Model file for the job. Use its own axes, mm. A direction names the side the tool comes from. Round coordinates to 2 decimals unless told otherwise and drop trailing zeros. Loops run counter-clockwise (first coordinate to the right, second up) from the corner with the lowest first, then second, coordinate; pieces in that order, holes last. Notation, with made-up numbers: M 9.25,14 L 68.25,14 A29 cw 68.25,45 Z; hole C 75.25,-17.75 d11. An arc over 180 degrees is marked long. Use a Markdown table: item, result. Add a question column.
Q1. Pin check, flat tips, straight feed: pin 1 (3 mm diameter, centred on x = -3, y = 5, fed in from +Z); pin 2 (0.5 mm diameter, centred on x = -1.5, y = 5, fed in from +Z); pin 3 (1.5 mm diameter, centred on x = -3.5, z = 1, fed in from -Y). Stop position of each tip, or through.
Q2. Mould opens along X. For faces 3 (the face through (0, 0, 0)), 4 (the face through (4, 4, 2.8)), 5 (the face through (-2.17, -9.76, 1.49)), 6 (the face through (4.65, -2.85, 2.75)) say: +X half, -X half, draft (parallel to the pull), parting line (faces both ways), or undercut.
Q3. Probe line 1 (Z direction, x = -2.75, y = 7.5); line 2 (Z direction, x = 0, y = 7.25); line 3 (Y direction, x = 0.25, z = 1.5). List the from-to ranges inside material, lowest first. Write a range as from..to.
Q4. Tool access for faces 1 (the face through (4, -5, 3)), 2 (the face through (0.6, 0.1, 2.7)): list every direction of +Z, -Z, +X, -X, +Y, -Y with a clear straight run to the whole face (end or side of a thin tool).
Q5. Cut at A-A (z = 1.4). Give the cut face in (x, y).
from build123d import *

# Parameters (mm, degrees)
F0_R      = 10
F1_DEPTH  = 3
F2_R      = 1
F4_DEPTH  = 0.5
F5_DEPTH  = 0.5
F7_DEPTH  = 0.2
F8_DEPTH  = 0.2
F10_DEPTH = 0.2


with BuildPart() as f1:
    # F0 (on Top) → F1 (new body)
    with BuildSketch(Plane.XY):
        Circle(F0_R)
    extrude(amount=F1_DEPTH)

    # F2
    f2_edges = [f1.edges().sort_by_distance(p)[0] for p in [
        (-10, 0, 3),
        (-10, 0, 0),
    ]]
    fillet(f2_edges, radius=F2_R)

    # F3 (on face) → F4 (cut)
    with BuildSketch(Plane.XY.offset(3)):
        with BuildLine():
            Line((2.6188242033, -3.3776305377), (6.8794322408, -0.6989099297))
            add(Edge.make_bspline(
                [(2.0379616312, 8.7662256639), (1.6297293118, 7.760927147), (0.7947254097, 5.7046759771), (-0.2158731788, 1.9761788849), (0.9164418768, 0.0642277289), (2.929304388, -0.6172304518), (5.6350925737, 0.7468103985), (6.5537268756, -0.2412183766), (6.8794322408, -0.6989099297)],
                knots=[0, 0, 0, 0, 0.1908238507, 0.3903136826, 0.5337501788, 0.6776846025, 0.8516922871, 0.9633032231, 0.9633032231, 0.9633032231, 0.9633032231], degree=3))
            ThreePointArc((2.0379616312, 8.7662256639), (0.0759866512, 8.9996792181), (-1.8896505536, 8.7993875233))
            Line((-1.8896505536, 8.7993875233), (-2.3143994622, 5.9643280692))
            add(Edge.make_bspline(
                [(-2.3143994622, 5.9643280692), (-2.5209566799, 4.5856267279), (-2.998613389, 1.3974263723), (-5.1744957464, -0.6070257438), (-5.3903894892, -1.7340637252), (-5.4123916936, -2.0398823468)],
                knots=[0.2414805871, 0.2414805871, 0.2414805871, 0.2414805871, 0.5458400785, 0.8012843993, 0.8955104519, 0.8955104519, 0.8955104519, 0.8955104519], degree=3))
            Line((-5.4123916936, -2.0398823468), (2.6188242033, -3.3776305377))
        make_face()
    extrude(amount=-F4_DEPTH, mode=Mode.SUBTRACT)

    # F3 (on face) → F5 (cut)
    with BuildSketch(Plane.XY.offset(3)):
        with BuildLine():
            Line((3.2604557928, -3.7864416372), (6.0787242837, -1.8852878129))
            Line((6.0787242837, -1.8852878129), (7.1935072074, -1.1658464236))
            add(Edge.make_bspline(
                [(6.8794322408, -0.6989099297), (6.9865215417, -0.8493952261), (7.0900143745, -1.0076208248), (7.1935072074, -1.1658464236)],
                knots=[0.9633032231, 0.9633032231, 0.9633032231, 0.9633032231, 1, 1, 1, 1], degree=3))
            Line((6.8794322408, -0.6989099297), (2.6188242033, -3.3776305377))
            Line((2.6188242033, -3.3776305377), (-5.4123916936, -2.0398823468))
            add(Edge.make_bspline(
                [(-5.4123916936, -2.0398823468), (-5.4367904701, -2.3790120105), (-5.4167044889, -2.720741879), (-5.3966185078, -3.0624717474)],
                knots=[0.8955104519, 0.8955104519, 0.8955104519, 0.8955104519, 1, 1, 1, 1], degree=3))
            Line((-5.3966185078, -3.0624717474), (2.5323872936, -4.2450306214))
            Line((2.5323872936, -4.2450306214), (3.2604557928, -3.7864416372))
        make_face()
    extrude(amount=-F5_DEPTH, mode=Mode.SUBTRACT)

    # F6 (on face) → F7 (join)
    with BuildSketch(Plane.XY.offset(2.5)):
        with BuildLine():
            add(Edge.make_bspline(
                [(-2.3842653189, 5.5020927108), (-2.400709991, 5.3951104015), (-2.4176575323, 5.2866589487), (-2.4352520085, 5.1770578662)],
                knots=[0.2746404016, 0.2746404016, 0.2746404016, 0.2746404016, 0.2971489273, 0.2971489273, 0.2971489273, 0.2971489273], degree=3))
            Line((-2.4352520085, 5.1770578662), (0.625273791, 4.9229885711))
            add(Edge.make_bspline(
                [(0.760314553, 5.3573187551), (0.7143347288, 5.2141615037), (0.6690819594, 5.0691118902), (0.625273791, 4.9229885711)],
                knots=[0.2034219896, 0.2034219896, 0.2034219896, 0.2034219896, 0.2264819887, 0.2264819887, 0.2264819887, 0.2264819887], degree=3))
            Line((0.760314553, 5.3573187551), (-2.3842653189, 5.5020927108))
        make_face()
    extrude(amount=F7_DEPTH)

    # F3 (on face) → F8 (cut)
    with BuildSketch(Plane.XY.offset(3)):
        with BuildLine():
            Line((-3.7310567152, -8.1901902169), (2.5323872936, -4.2450306214))
            Line((2.5323872936, -4.2450306214), (-5.3966185078, -3.0624717474))
            add(Edge.make_bspline(
                [(-5.4123916936, -2.0398823468), (-5.4367904701, -2.3790120105), (-5.4167044889, -2.720741879), (-5.3966185078, -3.0624717474)],
                knots=[0.8955104519, 0.8955104519, 0.8955104519, 0.8955104519, 1, 1, 1, 1], degree=3))
            add(Edge.make_bspline(
                [(-2.3143994622, 5.9643280692), (-2.5209566799, 4.5856267279), (-2.998613389, 1.3974263723), (-5.1744957464, -0.6070257438), (-5.3903894892, -1.7340637252), (-5.4123916936, -2.0398823468)],
                knots=[0.2414805871, 0.2414805871, 0.2414805871, 0.2414805871, 0.5458400785, 0.8012843993, 0.8955104519, 0.8955104519, 0.8955104519, 0.8955104519], degree=3))
            Line((-2.3143994622, 5.9643280692), (-1.8896505536, 8.7993875233))
            ThreePointArc((-1.8896505536, 8.7993875233), (-8.9475988677, 0.9697806466), (-3.7310567152, -8.1901902169))
        make_face()
        with BuildLine():
            add(Edge.make_bspline(
                [(6.8794322408, -0.6989099297), (6.9865215417, -0.8493952261), (7.0900143745, -1.0076208248), (7.1935072074, -1.1658464236)],
                knots=[0.9633032231, 0.9633032231, 0.9633032231, 0.9633032231, 1, 1, 1, 1], degree=3))
            Line((7.1935072074, -1.1658464236), (9, 0))
            ThreePointArc((9, 0), (7.0477533541, 5.5972468822), (2.0379616312, 8.7662256639))
            add(Edge.make_bspline(
                [(2.0379616312, 8.7662256639), (1.6297293118, 7.760927147), (0.7947254097, 5.7046759771), (-0.2158731788, 1.9761788849), (0.9164418768, 0.0642277289), (2.929304388, -0.6172304518), (5.6350925737, 0.7468103985), (6.5537268756, -0.2412183766), (6.8794322408, -0.6989099297)],
                knots=[0, 0, 0, 0, 0.1908238507, 0.3903136826, 0.5337501788, 0.6776846025, 0.8516922871, 0.9633032231, 0.9633032231, 0.9633032231, 0.9633032231], degree=3))
        make_face()
    extrude(amount=-F8_DEPTH, mode=Mode.SUBTRACT)

    # F9 (on face) → F10 (join)
    with BuildSketch(Plane.XY.offset(2.5)):
        Polygon((0.4235866599, 1.0353629961), (0.2137521335, 1.6472745719), (-0.5133344134, 1.4130915244), (-0.2446945873, 0.7603343111), align=None)
        Polygon((1.1939833379, 0.1412997616), (0.7390651665, 0.5554548462), (0.1189987625, 0.1596583386), (0.4858149623, -0.3592776484), align=None)
        Polygon((2.4212828624, -0.2853942997), (1.5963621816, -0.0867172381), (1.0029768368, -0.780917181), (1.7334064469, -1.1658464236), align=None)
    extrude(amount=F10_DEPTH)


solid = f1.part
Checked values:
| question | item | result |
|---|---|---|
| 1 | pin 1 | stops at z = 2.8 |
| 1 | pin 2 | stops at z = 2.7 |
| 1 | pin 3 | stops at y = -9.61 |
| 2 | face 3 | draft |
| 2 | face 4 | undercut |
| 2 | face 5 | parting line |
| 2 | face 6 | undercut |
| 3 | line 1 | z = 0..2.8 |
| 3 | line 2 | z = 0..2.5 |
| 3 | line 3 | y = -10..10 |
| 4 | face 1 | +Z, +X, -X, +Y, -Y |
| 4 | face 2 | +Z |
| 5 | outline | C 0,0 d20 |
